The listing builds one solid part. Answer for the finished solid, in the listing's coordinates (mm). Face numbers are marked on the shaded views. A direction names the side the tool comes from. Round coordinates to 2 decimals unless told otherwise and drop trailing zeros. Order: outer loops, then holes, each group sorted by start corner. A loop starts at its lowest first (then second) coordinate and runs counter-clockwise, first axis right, second up. Notation, with made-up numbers: M 46.25,1.5 L 104.25,1.5 A19 cw 104.25,28.5 Z; hole C -9.5,-27.75 d7. An arc over 180 degrees is marked long. Put each result on its own line as item: value. Start each with the question number.
1. Consider line 1 (Z direction, x = 19, y = 25); line 2 (X direction, y = 32, z = -6); line 3 (Y direction, x = 46, z = -2.5). Determine where each line is inside the solid, lowest interval first.
2. The mould has two halves that part along Z. Classify the marked faces 1, 2 and 3: +Z half, -Z half, draft (parallel to the pull), parting line (faces both ways), or undercut.
3. Each of these flat-tipped pins is pushed along its axis until it touches: pin 1 Ø2 at (y, z) = (205.5, -17) entering from +X; pin 2 Ø3.5 at (x, z) = (6.35, -44.45) entering from -Y; pin 3 Ø2.5 at (x, z) = (19.05, -44.45) entering from -Y. Where does it stop, or does it pass through?
4. The part is cut by section D-D (y = 113.5). Give the vertices of the cut face in (x, z).
5. The part is cut by section C-C (z = -26). Give the vertices of the cut face in (x, y), then the cut area to 3 significant figures.
6. The part is cut by section B-B (x = 50.8). Give the vertices of the cut face in (y, z).
7. The part is cut by section A-A (y = 15.5). Give the vertices of the cut face in (x, z), then the cut area to 3 significant figures.
8. Which of the six approach directions +Z, -Z, +X, -X, +Y, -Y give full straight-line access (tool end or side, diameter ignored) to the marked faces 4 and 5?
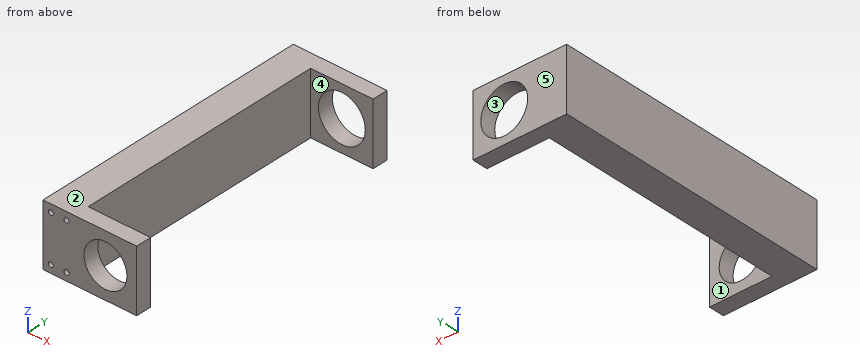
from build123d import *

# Parameters (mm, degrees)
SKETCH1_W                  = 76.2
SKETCH1_H                  = 50.8
BOSS_EXTRUDE1_DEPTH        = 228.6
SKETCH2_W                  = 50.8
SKETCH2_H                  = 203.2
CUT_EXTRUDE1_DEPTH         = 247.262136757
CUT_EXTRUDE2_REACH         = 248.262
SKETCH5_R                  = 19.05
CUT_EXTRUDE3_REACH         = 248.262
SKETCH8_R                  = 17.4625
F_10_32_TAPPED_HOLE1_D     = 4.0386
F_10_32_TAPPED_HOLE1_DEPTH = 42.0624
F_10_32_TAPPED_HOLE1_TIP   = 1.213317848


with BuildPart() as part:
    # Sketch1 → Boss-Extrude1 (new body)
    with BuildSketch(Plane(origin=(0, 0, 0), x_dir=(1, 0, 0), z_dir=(0, 1, 0))):
        with Locations((38.1, 25.4)):
            Rectangle(SKETCH1_W, SKETCH1_H)
    extrude(amount=BOSS_EXTRUDE1_DEPTH)

    # Sketch2 → Cut-Extrude1 (cut, through all)
    with BuildSketch(Plane.XY):
        with Locations((50.8, 114.3)):
            Rectangle(SKETCH2_W, SKETCH2_H)
    extrude(amount=-CUT_EXTRUDE1_DEPTH, mode=Mode.SUBTRACT)

    # Sketch5 → Cut-Extrude2 (cut, up to next)
    with BuildSketch(Plane(origin=(0, 228.6, 0), x_dir=(1, 0, 0), z_dir=(0, 1, 0)), mode=Mode.PRIVATE) as cut_extrude2_sk1:
        with Locations(Location((50.8, 25.4, 0), (0, 0, 270))):
            Circle(SKETCH5_R)
    cut_extrude2_tool1 = extrude(cut_extrude2_sk1.sketch, amount=-CUT_EXTRUDE2_REACH, mode=Mode.PRIVATE) & part.part
    add(cut_extrude2_tool1.solids().sort_by_distance((50.8, 228.6, -25.4))[0], mode=Mode.SUBTRACT)

    # Sketch8 → Cut-Extrude3 (cut, up to next)
    with BuildSketch(Plane.XZ, mode=Mode.PRIVATE) as cut_extrude3_sk1:
        with Locations(Location((50.8, -25.4, 0), (0, 0, 270))):
            Circle(SKETCH8_R)
    cut_extrude3_tool1 = extrude(cut_extrude3_sk1.sketch, amount=-CUT_EXTRUDE3_REACH, mode=Mode.PRIVATE) & part.part
    add(cut_extrude3_tool1.solids().sort_by_distance((50.8, 0, -25.4))[0], mode=Mode.SUBTRACT)

    # #10-32 Tapped Hole1
    with Locations(Plane(origin=(0, 0, 0), x_dir=(-1, 0, 0), z_dir=(0, -1, 0))):
        with Locations((-6.35, 44.45), (-19.05, 44.45), (-6.35, 6.35), (-19.05, 6.35)):
            Hole(F_10_32_TAPPED_HOLE1_D / 2, depth=F_10_32_TAPPED_HOLE1_DEPTH)
            with Locations((0, 0, -(F_10_32_TAPPED_HOLE1_DEPTH + F_10_32_TAPPED_HOLE1_TIP / 2))):  # 118° drill point
                Cone(0, F_10_32_TAPPED_HOLE1_D / 2, F_10_32_TAPPED_HOLE1_TIP, mode=Mode.SUBTRACT)


solid = part.part
Resolved:
1. line 1: -50.8 to -46.47, -42.43 to -8.37, -4.33 to 0
1. line 2: 0 to 4.36, 8.34 to 17.06, 21.04 to 25.4
1. line 3: 0 to 12.7, 215.9 to 228.6
2. face 1: draft
2. face 2: +Z half
2. face 3: undercut
3. pin 1: x = 25.4
3. pin 2: y = 42.22
3. pin 3: y = 42.52
4. outline: M 0,-50.8 L 25.4,-50.8 L 25.4,0 L 0,0 Z
5. outline: M 0,0 L 33.35,0 L 33.35,12.7 L 25.4,12.7 L 25.4,215.9 L 31.76,215.9 L 31.76,228.6 L 0,228.6 Z; M 68.25,0 L 76.2,0 L 76.2,12.7 L 68.25,12.7 Z; M 69.84,215.9 L 76.2,215.9 L 76.2,228.6 L 69.84,228.6 Z
5. area: 6,170 mm2
6. outline: M 0,-50.8 L 12.7,-50.8 L 12.7,-42.86 L 0,-42.86 Z; M 0,-7.94 L 12.7,-7.94 L 12.7,0 L 0,0 Z; M 215.9,-50.8 L 228.6,-50.8 L 228.6,-44.45 L 215.9,-44.45 Z; M 215.9,-6.35 L 228.6,-6.35 L 228.6,0 L 215.9,0 Z
7. outline: M 0,-50.8 L 25.4,-50.8 L 25.4,0 L 0,0 Z; hole C 6.35,-44.45 d4.04; hole C 6.35,-6.35 d4.04; hole C 19.05,-44.45 d4.04; hole C 19.05,-6.35 d4.04
7. area: 1,240 mm2
8. face 4: +Z, -Z, +X
8. face 5: +Z, -Z, +X, -X, +Y
